Part model, mm, in its own coordinate system. A direction names the side the tool comes from. Give positions to 0.01 mm unless a question says otherwise; leave off trailing zeros. Write each loop counter-clockwise with the first axis right and the second up, starting at its lowest first coordinate (ties: lowest second). Pieces come first, ordered by that corner, then holes.
from build123d import *

# Parameters (mm, degrees)
BOSS_EXTRUDE1_DEPTH = 7
CUT_EXTRUDE1_DEPTH  = 5


with BuildPart() as part:
    # Sketch1 → Revolve1 (revolve)
    with BuildSketch(Plane.XY):
        with BuildLine():
            Line((-4.75, 5.5), (-4.75, 7.5))
            Line((-4.75, 7.5), (5.25, 3.755937126))
            Line((5.25, 3.755937126), (5.25, 7.5))
            Line((5.25, 7.5), (10.25, 7.5))
            Line((10.25, 7.5), (10.25, 6.5))
            ThreePointArc((10.25, 6.5), (11.75, 5), (10.25, 3.5))
            Line((10.25, 3.5), (10.25, 2.5))
            Line((10.25, 2.5), (10.25, 0))
            Line((10.25, 0), (7.25, 0))
            Line((7.25, 0), (7.25, 2))
            Line((7.25, 2), (0.25, 2))
            Line((0.25, 2), (0.25, 3.75))
            Line((0.25, 3.75), (-4.75, 5.5))
        make_face()
    revolve(axis=Axis((-16.375, 0, 0), (1, 0, 0)))

    # Sketch2 → Boss-Extrude1 (add)
    with BuildSketch(Plane.ZY.offset(-0.25)):
        with BuildLine():
            Line((1.1, 1.670329309), (1.1, -1.670329309))
            ThreePointArc((1.1, -1.670329309), (2, 0), (1.1, 1.670329309))
        make_face()
    extrude(amount=-BOSS_EXTRUDE1_DEPTH)

    # Sketch3 → Cut-Extrude1 (cut)
    with BuildSketch(Plane(origin=(10.25, 0, 0), x_dir=(0, 0, -1), z_dir=(1, 0, 0))):
        with BuildLine():
            ThreePointArc((-4.550626724, -5.96169409), (-4.303857188, -5.269948975), (-4.596194072, -4.596194084))
            ThreePointArc((-4.596194072, -4.596194084), (-5.269948967, -4.303857188), (-5.96169409, -4.550626724))
            ThreePointArc((-5.96169409, -4.550626724), (-5.303300859, -5.303300859), (-4.550626724, -5.96169409))
        make_face()
        with BuildLine():
            ThreePointArc((-1.922789333, -7.249336603), (-1.959523399, -6.515812848), (-2.487442279, -6.005216974))
            ThreePointArc((-2.487442279, -6.005216974), (-3.221783135, -5.992967721), (-3.766437695, -6.485672447))
            ThreePointArc((-3.766437695, -6.485672447), (-2.870125743, -6.929096494), (-1.922789333, -7.249336603))
        make_face()
        with BuildLine():
            ThreePointArc((0.997775303, -7.433333333), (0.683130051, -6.769703257), (0, -6.5))
            ThreePointArc((0, -6.5), (-0.683130051, -6.769703257), (-0.997775303, -7.433333333))
            ThreePointArc((-0.997775303, -7.433333333), (0, -7.5), (0.997775303, -7.433333333))
        make_face()
        with BuildLine():
            ThreePointArc((3.766437695, -6.485672447), (3.221782808, -5.992967599), (2.487441634, -6.005217241))
            ThreePointArc((2.487441634, -6.005217241), (1.959523255, -6.515813166), (1.922789333, -7.249336603))
            ThreePointArc((1.922789333, -7.249336603), (2.870125743, -6.929096494), (3.766437695, -6.485672447))
        make_face()
        with BuildLine():
            ThreePointArc((5.96169409, -4.550626724), (5.269948971, -4.303857188), (4.596194077, -4.596194078))
            ThreePointArc((4.596194077, -4.596194078), (4.303857188, -5.269948971), (4.550626724, -5.96169409))
            ThreePointArc((4.550626724, -5.96169409), (5.303300859, -5.303300859), (5.96169409, -4.550626724))
        make_face()
        with BuildLine():
            ThreePointArc((7.249336603, -1.922789333), (6.51581242, -1.959523594), (6.005216614, -2.487443148))
            ThreePointArc((6.005216614, -2.487443148), (5.992967887, -3.221783575), (6.485672447, -3.766437695))
            ThreePointArc((6.485672447, -3.766437695), (6.929096494, -2.870125743), (7.249336603, -1.922789333))
        make_face()
        with BuildLine():
            ThreePointArc((6.485672447, 3.766437695), (5.992967893, 3.221783593), (6.0052166, 2.487443183))
            ThreePointArc((6.0052166, 2.487443183), (6.515812403, 1.959523601), (7.249336603, 1.922789333))
            ThreePointArc((7.249336603, 1.922789333), (6.929096494, 2.870125743), (6.485672447, 3.766437695))
        make_face()
        with BuildLine():
            ThreePointArc((7.433333333, 0.997775303), (6.769703257, 0.683130051), (6.5, 0))
            ThreePointArc((6.5, 0), (6.769703257, -0.683130051), (7.433333333, -0.997775303))
            ThreePointArc((7.433333333, -0.997775303), (7.483314774, -0.5), (7.5, 0))
            ThreePointArc((7.5, 0), (7.483314774, 0.5), (7.433333333, 0.997775303))
        make_face()
        with BuildLine():
            ThreePointArc((4.550626724, 5.96169409), (4.303857188, 5.269948971), (4.596194078, 4.596194078))
            ThreePointArc((4.596194078, 4.596194078), (5.269948971, 4.303857188), (5.96169409, 4.550626724))
            ThreePointArc((5.96169409, 4.550626724), (5.303300859, 5.303300859), (4.550626724, 5.96169409))
        make_face()
        with BuildLine():
            ThreePointArc((1.922789333, 7.249336603), (1.959523233, 6.515813213), (2.487441538, 6.005217281))
            ThreePointArc((2.487441538, 6.005217281), (3.221782759, 5.99296758), (3.766437695, 6.485672447))
            ThreePointArc((3.766437695, 6.485672447), (2.870125743, 6.929096494), (1.922789333, 7.249336603))
        make_face()
        with BuildLine():
            ThreePointArc((-0.997775303, 7.433333333), (-0.683130051, 6.769703257), (0, 6.5))
            ThreePointArc((0, 6.5), (0.683130051, 6.769703257), (0.997775303, 7.433333333))
            ThreePointArc((0.997775303, 7.433333333), (0, 7.5), (-0.997775303, 7.433333333))
        make_face()
        with BuildLine():
            ThreePointArc((-6.005216971, -2.487442288), (-6.515812844, -1.959523401), (-7.249336603, -1.922789333))
            ThreePointArc((-7.249336603, -1.922789333), (-6.929096494, -2.870125743), (-6.485672447, -3.766437695))
            ThreePointArc((-6.485672447, -3.766437695), (-5.992967723, -3.221783139), (-6.005216971, -2.487442288))
        make_face()
        with BuildLine():
            ThreePointArc((-7.433333333, 0.997775303), (-7.5, 0), (-7.433333333, -0.997775303))
            ThreePointArc((-7.433333333, -0.997775303), (-6.769703257, -0.683130051), (-6.5, 0))
            ThreePointArc((-6.5, 0), (-6.769703257, 0.683130051), (-7.433333333, 0.997775303))
        make_face()
        with BuildLine():
            ThreePointArc((-7.249336603, 1.922789333), (-6.515812818, 1.959523413), (-6.005216949, 2.487442341))
            ThreePointArc((-6.005216949, 2.487442341), (-5.992967733, 3.221783166), (-6.485672447, 3.766437695))
            ThreePointArc((-6.485672447, 3.766437695), (-6.929096494, 2.870125743), (-7.249336603, 1.922789333))
        make_face()
        with BuildLine():
            ThreePointArc((-5.96169409, 4.550626724), (-5.269948974, 4.303857188), (-4.596194082, 4.596194074))
            ThreePointArc((-4.596194082, 4.596194074), (-4.303857188, 5.269948968), (-4.550626724, 5.96169409))
            ThreePointArc((-4.550626724, 5.96169409), (-5.303300859, 5.303300859), (-5.96169409, 4.550626724))
        make_face()
        with BuildLine():
            ThreePointArc((-3.766437695, 6.485672447), (-3.221783319, 5.992967791), (-2.487442643, 6.005216823))
            ThreePointArc((-2.487442643, 6.005216823), (-1.959523481, 6.515812669), (-1.922789333, 7.249336603))
            ThreePointArc((-1.922789333, 7.249336603), (-2.870125743, 6.929096494), (-3.766437695, 6.485672447))
        make_face()
    extrude(amount=-CUT_EXTRUDE1_DEPTH, mode=Mode.SUBTRACT)


solid = part.part
1) Saw through at C-C (x = 2). Write the cut outline in (y, z), and give its area (3 significant figures).
Check result:
outline: circle Ø9.95 at (0, 0); hole (-1.67, 1.1) arc R2 ccw (long way) to (1.67, 1.1) - close
area: 67.2 mm2
2) Mould opens along Z. For faces 1 (the cylindrical face through (4, 0, -2)), 2 (the flat face through (10.25, 6.8, 1.3)), 3 (the cylindrical face through (7.785, 1.457, -7.357)) say: +Z half, -Z half, draft (parallel to the pull), parting line (faces both ways), or undercut.
Check result:
face 1: undercut
face 2: draft
face 3: -Z half
3) Saw through at B-B (y = 6.25). State how many separate pieces and enclosed holes the cut face has, and give its area (3 significant figures).
Check result:
separate pieces: 4
enclosed holes: 0
area: 47.2 mm2
4) Drill centre lines: L1, parallel to Y at x = 5.5, z = 0; L2, parallel to Y at x = 5.5, z = 6.25; L3, parallel to X at y = -0.5, z = 2.25. Where is each one in solid material? Low to high.
Check result:
L1: y = -6.5 to -2, 2 to 6.5
L2: y = -4.15 to -3.6, -2.14 to 2.14, 3.6 to 4.15
L3: x = 0.25 to 10.25
5) 3-axis set-ups, long thin cutter, end or side, ignore diameter. For faces 4 (the flat face through (5.25, -3, -3)), 5 (the flat face through (10.25, 0, 0)), 6 (the flat face through (10.25, -6.8, -1.3)): which of +Z, -Z, +X, -X, +Y, -Y reach the whole face in a straight line?
Check result:
face 4: none
face 5: +X
face 6: -Z, +X, -Y
6) Flat gauge pins, fed straight in: P1, Ø6, axis at x = 8.5, y = 1, coming from the +Z side; P2, Ø0.6, axis at y = 3.5, z = 6, coming from the +X side; P3, Ø4, axis at x = 5.5, z = 2, coming from the -Y side. Where does each tip first touch, or does it go through?
Check result:
P1: stops at z = 7.43
P2: stops at x = 10.25
P3: stops at y = -7.43
7) Saw through at A-A (x = -1.25). Write the cut outline in (y, z) (3 decimals), and give its area (3 significant figures).
Check result:
outline: circle Ø12.379 at (0, 0); hole circle Ø8.55 at (0, 0)
area: 62.9 mm2
